The model under review builds one solid part; all positions refer to its coordinate system, in mm. A direction names the side the tool comes from. Round coordinates to 2 decimals unless told otherwise and drop trailing zeros. Write each loop counter-clockwise with the first axis right and the second up, starting at its lowest first coordinate (ties: lowest second). Pieces come first, ordered by that corner, then holes. Notation, with made-up numbers: M 10.25,-29.5 L 63.25,-29.5 A15 ccw 63.25,-1.5 Z; hole C 19.25,20 d9. An arc over 180 degrees is marked long. Write item = value, one per line. Start each with the question number.
Item 1: Tool access review of faces 4 (the flat face through (-66, -228, 90.932)), 5 (the flat face through (-57, -350, 61)), 6 (the flat face through (-64.879, -173, 79)), 7 (the flat face through (-58, -185, -74.558)), 8 (the flat face through (-44.879, -185, 98)): name each direction out of +Z, -Z, +X, -X, +Y, -Y from which nothing blocks a thin tool from reaching the whole face with its end or side.
Item 2: Take a section at A-A, the plane z = 70.5. Give the boundary of the cut face in (x, y), plus the area to 3 significant figures.
Item 3: The part is to be moulded in two halves that separate along Z. For faces 1 (the flat face through (-58, -185, 275.442)), 2 (the flat face through (-57.2, -362.68, 43.61)), 3 (the flat face through (-58, -375, -8)), say which applies: +Z half, -Z half, draft (parallel to the pull), parting line (faces both ways), or undercut.
Item 4: To check wall thickness, follow line 1 along Z through (x, y) = (-68.25, -318.5); line 2 along Y through (x, z) = (-61.75, 71.5); line 3 along Y through (x, z) = (-49, 54.5). State the ranges of each line that lie inside material, in increasing order.
Item 5: For pin 1 Ø4 at (x, z) = (-58, 104) entering from +Y, flat-tipped, find the tip position at first contact; note if it passes through.
from build123d import *

# Parameters (mm, degrees)
F0_W     = 25
F0_H     = 350
F1_DEPTH = 375
F3_DEPTH = 25
F4_W     = 350
F4_H     = 25
F5_DEPTH = 5


with BuildPart() as f1:
    # F0 (on Front) → F1 (new body)
    with BuildSketch(Plane.XZ):
        with Locations((-57.378992, 100.442262)):
            Rectangle(F0_W, F0_H)
    extrude(amount=F1_DEPTH)

    # F2 (on face) → F3 (cut)
    with BuildSketch(Plane.YZ.offset(-44.878992)):
        Polygon((-375, 90.931553), (-375, 55.931553), (-350, 30.931553), (-350, 90.931553), align=None)
    extrude(amount=-F3_DEPTH, mode=Mode.SUBTRACT)

    # F4 (on face) → F5 (cut)
    with BuildSketch(Plane(origin=(-69.878992, 0, 0), x_dir=(0, -1, 0), z_dir=(-1, 0, 0))):
        with Locations((175, 78.431553)):
            Rectangle(F4_W, F4_H)
    extrude(amount=-F5_DEPTH, mode=Mode.SUBTRACT)


solid = f1.part
Response values:
q1.face_4 = -X, -Y
q1.face_5 = +X, -X
q1.face_6 = -X, +Y, -Y
q1.face_7 = -Z, +X, -X, +Y, -Y
q1.face_8 = +Z, -Z, +X, +Y, -Y
q2.outline = M -64.88,-350 L -44.88,-350 L -44.88,0 L -64.88,0 Z
q2.area = 7,000 mm2
q3.face_1 = +Z half
q3.face_2 = undercut
q3.face_3 = draft
q4.line_1 = -74.56 to 65.93, 90.93 to 275.44
q4.line_2 = -350 to 0
q4.line_3 = -375 to -373.57, -350 to 0
q5.pin_1 = 0
